Input: part model. Units: mm. Frame: model coordinates. A direction names the side the tool comes from. Round coordinates to 2 decimals unless told otherwise and drop trailing zeros. Write each loop counter-clockwise with the first axis right and the second up, starting at its lowest first coordinate (ties: lowest second). Pieces come first, ordered by that corner, then holes. Notation, with made-up numbers: (-36, 84) -> (16, 84) arc R21 ccw to (16, 97) -> close; hole circle Ø4 at (60.25, 38). An arc over 180 degrees is marked (long way). Write item = value, one per line.
```python
from build123d import *

# Parameters (mm, degrees)
F1_DEPTH = 10.16
F3_DEPTH = 5.08
F2_R     = 2.0763624022
F2_R_2   = 1.0345950723
F2_R_3   = 1.5897491602
F2_R_4   = 2.2416189492
F2_R_5   = 1.8002482779
F2_R_6   = 1.0905586669
F2_R_7   = 1.5614432183
F2_R_8   = 2.0977283719
F2_R_9   = 4.6843284207
F4_DEPTH = 4.572
F5_DEPTH = 7.62
F6_DEPTH = 0.762


# Not quite as in the source:
# - the program builds the solid bodies; features that only make, move or delete a surface that nothing else refers to are left out


with BuildPart() as f1:
    # F0 (on Top) → F1 (new body)
    with BuildSketch(Plane.XY):
        Polygon((47.8064281952, 65.5864290789), (-2.9935718048, 65.5864290789), (-2.9935718048, -10.6135709211), (-53.7935718048, -10.6135709211), (-53.7935718048, -61.4135709211), (47.8064281952, -61.4135709211), align=None)
    extrude(amount=F1_DEPTH)

    # F2 (on face) → F3 (cut)
    with BuildSketch(Plane.XY.offset(10.16)):
        with BuildLine():
            add(Edge.make_bspline(
                [(-47.8390082717, -23.6159972847), (-48.3000888755, -24.195855305), (-47.0430336613, -26.5169441972), (-43.1187716407, -22.9708090315), (-47.273269231, -22.904520121), (-47.8390082717, -23.6159972847)],
                knots=[0, 0, 0, 0, 0.2953373029, 0.6376255235, 1, 1, 1, 1], degree=3))
        make_face()
        with BuildLine():
            add(Edge.make_bspline(
                [(-45.2185384929, -37.5918187201), (-44.8986430919, -37.0721449164), (-46.7922945126, -35.0952494412), (-49.3003635487, -38.0785129033), (-45.5819638525, -38.1822074482), (-45.2185384929, -37.5918187201)],
                knots=[0, 0, 0, 0, 0.3255188332, 0.6301859964, 1, 1, 1, 1], degree=3))
        make_face()
        with BuildLine():
            add(Edge.make_bspline(
                [(-46.8684621155, -50.3168739378), (-46.3188154002, -50.6408562263), (-45.7691686849, -50.9648385147), (-45.2195219696, -51.2888208032)],
                knots=[0, 0, 0, 0, 1.9140753157, 1.9140753157, 1.9140753157, 1.9140753157], degree=3))
            add(Edge.make_bspline(
                [(-46.8684621155, -50.3168739378), (-47.7573276365, -50.4835154275), (-49.3321466932, -50.7787571568), (-47.6954089883, -52.20576886), (-46.1489762809, -51.633045446), (-45.2195219696, -51.2888208032)],
                knots=[0, 0, 0, 0, 0.340798916, 0.6037995791, 1, 1, 1, 1], degree=3))
        make_face()
    extrude(amount=-F3_DEPTH, mode=Mode.SUBTRACT)

    # F2 (on face) → F4 (cut)
    with BuildSketch(Plane.XY.offset(10.16)):
        with BuildLine():
            Line((0, -14.423571527), (-49.5299994946, -14.423571527))
            Line((-49.5299994946, -14.423571527), (-49.5299994946, -57.694286108))
            Line((-49.5299994946, -57.694286108), (12.2464280576, -57.694286108))
            add(Edge.make_bspline(
                [(12.2464280576, -57.694286108), (11.03689249, -55.1284041984), (8.8262402555, -50.4387756091), (16.830567108, -50.610538154), (11.543684395, -41.4140537661), (24.3541608342, -47.2929208414), (18.6630964396, -34.0142041282), (32.3027129745, -41.5037229838), (28.8060301659, -27.219324679), (39.7417437225, -32.4995208739), (41.581315462, -27.9924233376), (42.4542874098, -25.8535724133)],
                knots=[0, 0, 0, 0, 0.1112734122, 0.2033729508, 0.3034169687, 0.4180959772, 0.5306525521, 0.6520560864, 0.7731880867, 0.8923660146, 1, 1, 1, 1], degree=3))
            Line((42.4542874098, -25.8535724133), (42.4542874098, 61.7764294147))
            Line((42.4542874098, 61.7764294147), (0, 61.7764294147))
            Line((0, 61.7764294147), (0, -14.423571527))
        make_face()
        with BuildLine():
            add(Edge.make_bspline(
                [(-46.8684621155, -50.3168739378), (-47.7573276365, -50.4835154275), (-49.3321466932, -50.7787571568), (-47.6954089883, -52.20576886), (-46.1489762809, -51.633045446), (-45.2195219696, -51.2888208032)],
                knots=[0, 0, 0, 0, 0.340798916, 0.6037995791, 1, 1, 1, 1], degree=3))
            add(Edge.make_bspline(
                [(-46.8684621155, -50.3168739378), (-46.3188154002, -50.6408562263), (-45.7691686849, -50.9648385147), (-45.2195219696, -51.2888208032)],
                knots=[0, 0, 0, 0, 1.9140753157, 1.9140753157, 1.9140753157, 1.9140753157], degree=3))
        make_face(mode=Mode.SUBTRACT)
        with BuildLine():
            add(Edge.make_bspline(
                [(-45.2185384929, -37.5918187201), (-44.8986430919, -37.0721449164), (-46.7922945126, -35.0952494412), (-49.3003635487, -38.0785129033), (-45.5819638525, -38.1822074482), (-45.2185384929, -37.5918187201)],
                knots=[0, 0, 0, 0, 0.3255188332, 0.6301859964, 1, 1, 1, 1], degree=3))
        make_face(mode=Mode.SUBTRACT)
        with BuildLine():
            add(Edge.make_bspline(
                [(-47.8390082717, -23.6159972847), (-48.3000888755, -24.195855305), (-47.0430336613, -26.5169441972), (-43.1187716407, -22.9708090315), (-47.273269231, -22.904520121), (-47.8390082717, -23.6159972847)],
                knots=[0, 0, 0, 0, 0.2953373029, 0.6376255235, 1, 1, 1, 1], degree=3))
        make_face(mode=Mode.SUBTRACT)
        with Locations((2.6250390802, 47.6025752723)):
            Circle(F2_R, mode=Mode.SUBTRACT)
        with Locations((6.2461188063, 49.3268966675)):
            Circle(F2_R_2, mode=Mode.SUBTRACT)
        with Locations((3.4872009419, 52.4306818843)):
            Circle(F2_R_3, mode=Mode.SUBTRACT)
        with Locations((3.6596332211, 58.1209473312)):
            Circle(F2_R_4, mode=Mode.SUBTRACT)
        with Locations((7.9704420641, 53.8101382554)):
            Circle(F2_R_5, mode=Mode.SUBTRACT)
        with Locations((11.2466607243, 55.3620308638)):
            Circle(F2_R_6, mode=Mode.SUBTRACT)
        with Locations((10.0396340713, 59.1555424035)):
            Circle(F2_R_7, mode=Mode.SUBTRACT)
        with Locations((15.3850372881, 59.1555424035)):
            Circle(F2_R_8, mode=Mode.SUBTRACT)
        with Locations((33.3180055022, 52.6031143963)):
            Circle(F2_R_9, mode=Mode.SUBTRACT)
        with BuildLine():
            add(Edge.make_bspline(
                [(12.2464280576, -57.694286108), (11.03689249, -55.1284041984), (8.8262402555, -50.4387756091), (16.830567108, -50.610538154), (11.543684395, -41.4140537661), (24.3541608342, -47.2929208414), (18.6630964396, -34.0142041282), (32.3027129745, -41.5037229838), (28.8060301659, -27.219324679), (39.7417437225, -32.4995208739), (41.581315462, -27.9924233376), (42.4542874098, -25.8535724133)],
                knots=[0, 0, 0, 0, 0.1112734122, 0.2033729508, 0.3034169687, 0.4180959772, 0.5306525521, 0.6520560864, 0.7731880867, 0.8923660146, 1, 1, 1, 1], degree=3))
            Line((12.2464280576, -57.694286108), (42.4542874098, -57.694286108))
            Line((42.4542874098, -57.694286108), (42.4542874098, -25.8535724133))
        make_face()
    extrude(amount=-F4_DEPTH, mode=Mode.SUBTRACT)

    # F5 (cut): a face of the model
    f5_faces = [f1.faces().sort_by_distance(p)[0] for p in [
        (33.3180055022, 52.6031143963, 10.16),
    ]]
    extrude(f5_faces, amount=-F5_DEPTH, mode=Mode.SUBTRACT)

    # F2 (on face) → F6 (cut)
    with BuildSketch(Plane.XY.offset(10.16)):
        with BuildLine():
            add(Edge.make_bspline(
                [(12.2464280576, -57.694286108), (11.03689249, -55.1284041984), (8.8262402555, -50.4387756091), (16.830567108, -50.610538154), (11.543684395, -41.4140537661), (24.3541608342, -47.2929208414), (18.6630964396, -34.0142041282), (32.3027129745, -41.5037229838), (28.8060301659, -27.219324679), (39.7417437225, -32.4995208739), (41.581315462, -27.9924233376), (42.4542874098, -25.8535724133)],
                knots=[0, 0, 0, 0, 0.1112734122, 0.2033729508, 0.3034169687, 0.4180959772, 0.5306525521, 0.6520560864, 0.7731880867, 0.8923660146, 1, 1, 1, 1], degree=3))
            Line((12.2464280576, -57.694286108), (42.4542874098, -57.694286108))
            Line((42.4542874098, -57.694286108), (42.4542874098, -25.8535724133))
        make_face()
    extrude(amount=-F6_DEPTH, mode=Mode.SUBTRACT)


solid = f1.part
```
1) Cut plane C-C (x = -36). Return the cut outline in (y, z), and give its area (3 significant figures).
Solutions:
outline = (-61.41, 0) -> (-10.61, 0) -> (-10.61, 10.16) -> (-14.42, 10.16) -> (-14.42, 5.59) -> (-57.69, 5.59) -> (-57.69, 10.16) -> (-61.41, 10.16) -> close
area = 318 mm^2
2) Access query for faces 1 (the face through (-2.994, 28, 5)), 2 (the face through (33, 53, 2.54)), 3 (the face through (8, 54, 10.16)). Directions: +Z, -Z, +X, -X, +Y, -Y. A direction counts if a zero-diameter tool reaches every point of the face in a straight line with its end or side. Return the directions, or none.
Solutions:
face_1 = +Z, -Z, -X, +Y
face_2 = +Z
face_3 = +Z, +X, -X, +Y, -Y
3) Cut plane B-B (z = 7.75). Count the separate pieces of the cut face and the enclosed holes in it, and give its area (3 significant figures).
Solutions:
separate_pieces = 9
enclosed_holes = 1
area = 1,890 mm^2
4) First-contact query: P1, Ø1, axis at x = -46.5, y = -37, coming from the +Z side; P2, Ø2, axis at y = 25.5, z = 4.5, coming from the -X side; P3, Ø6, axis at x = -31, z = 1.5, coming from the +Y side. Flat tips, straight axial feed; report the tip coordinate or a pass-through.
Solutions:
P1 = 5.08
P2 = -2.99
P3 = -10.61
5) Cut plane D-D (x = 35.5). Return the cut outline in (y, z), and give its area (3 significant figures).
Solutions:
outline = (-61.41, 0) -> (65.59, 0) -> (65.59, 10.16) -> (61.78, 10.16) -> (61.78, 5.59) -> (56.75, 5.59) -> (56.75, 2.54) -> (48.46, 2.54) -> (48.46, 5.59) -> (-57.69, 5.59) -> (-57.69, 10.16) -> (-61.41, 10.16) -> close
area = 719 mm^2
6) Cut plane A-A (y = 36.5). Return the cut outline in (x, z), and give its area (3 significant figures).
Solutions:
outline = (-2.99, 0) -> (47.81, 0) -> (47.81, 10.16) -> (42.45, 10.16) -> (42.45, 5.59) -> (0, 5.59) -> (0, 10.16) -> (-2.99, 10.16) -> close
area = 322 mm^2
7) Line query: L1, parallel to Y at x = -39, z = 8.25; L2, parallel to Y at x = 19, z = 8; L3, parallel to X at y = 46.5, z = 9.25. Output: solid intervals per line, ascending. Write a range as from..to.
Solutions:
L1 = -61.41..-57.69, -14.42..-10.61
L2 = -61.41..-57.69, 61.78..65.59
L3 = -2.99..0, 0.87..4.38, 42.45..47.81
